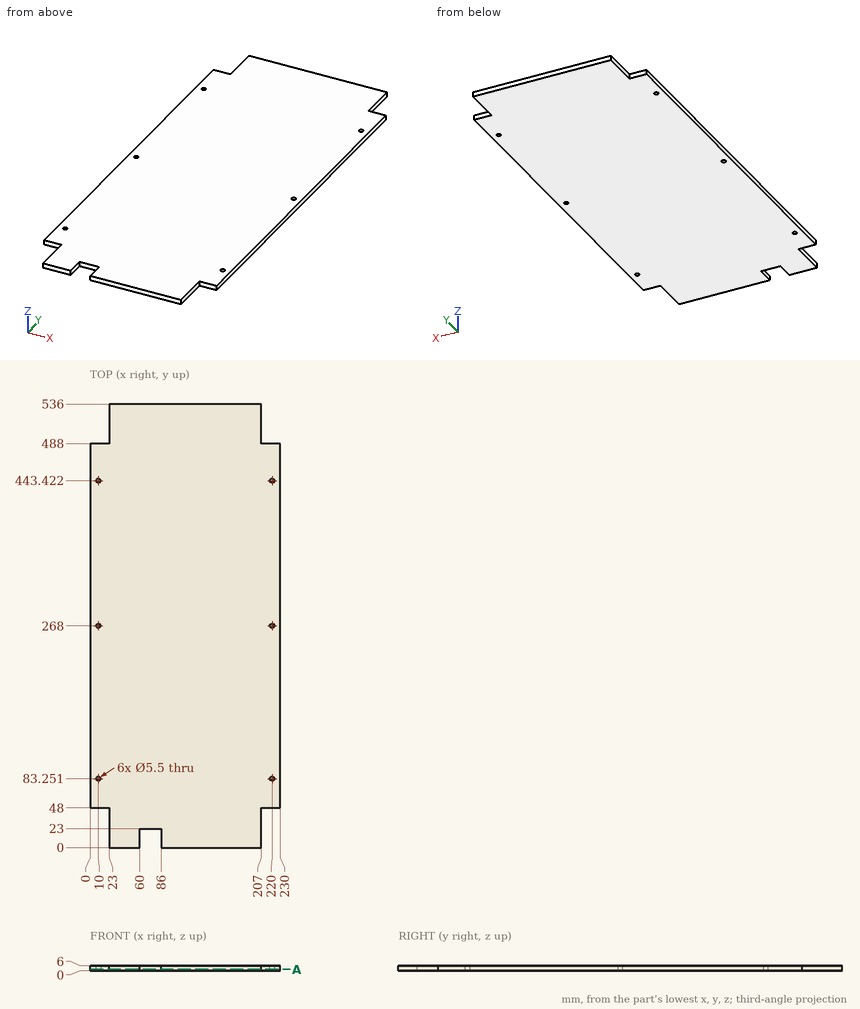
Design review of the part shown in the three views and the two pictorial views. Dimensions are in mm from the part's minimum x, y and z. Give positions to 0.01 mm unless a question says otherwise; leave off trailing zeros. Order: outer loops, then holes, each group sorted by start corner. A loop starts at its lowest first (then second) coordinate and runs counter-clockwise, first axis right, second up. Notation, with made-up numbers: M 72.5,-4.75 L 120.5,-4.75 A21 ccw 120.5,10.25 Z; hole C -39.5,33 d4. An arc over 180 degrees is marked long. Answer in a Markdown table with one row per item. Add a question column.
(1) For pin 1 (3 mm diameter, centred on y = 512.5, z = 4, fed in from -X); pin 2 (5 mm diameter, centred on x = 220, y = 83.25, fed in from +Z); pin 3 (3 mm diameter, centred on x = 221.5, z = 2, fed in from -Y); pin 4 (1.8 mm diameter, centred on y = 23, z = 2, fed in from +X), all flat-tipped, find the tip position at first contact; note any pin that passes through.
(2) Consider section A-A on z = 1.5. State the section outline as (x, y) points, and give its area (3 significant figures).
(3) Wall thickness on probe 1 along Y at (x, z) = (220, 1.55); probe 2 along Y at (x, z) = (219, 4.15) (1 decimal); probe 3 along X at (y, z) = (23.5, 1.9): over which ranges is each line inside the solid? List them lowest first. Write a range as [from, to].
Evaluation:
| question | item | result |
|---|---|---|
| 1 | pin 1 | stops at x = 23 |
| 1 | pin 2 | passes through |
| 1 | pin 3 | stops at y = 48 |
| 1 | pin 4 | stops at x = 207 |
| 2 | outline | M 0,48 L 23,48 L 23,0 L 60,0 L 60,23 L 86,23 L 86,0 L 207,0 L 207,48 L 230,48 L 230,488 L 207,488 L 207,536 L 23,536 L 23,488 L 0,488 Z; hole C 10,83.25 d5.5; hole C 10,268 d5.5; hole C 10,443.42 d5.5; hole C 220,83.25 d5.5; hole C 220,268 d5.5; hole C 220,443.42 d5.5 |
| 2 | area | 118,000 mm^2 |
| 3 | probe 1 | y = [48, 80.5], [86, 265.25], [270.75, 440.67], [446.17, 488] |
| 3 | probe 2 | y = [48, 80.7], [85.8, 265.4], [270.6, 440.9], [446, 488] |
| 3 | probe 3 | x = [23, 207] |
